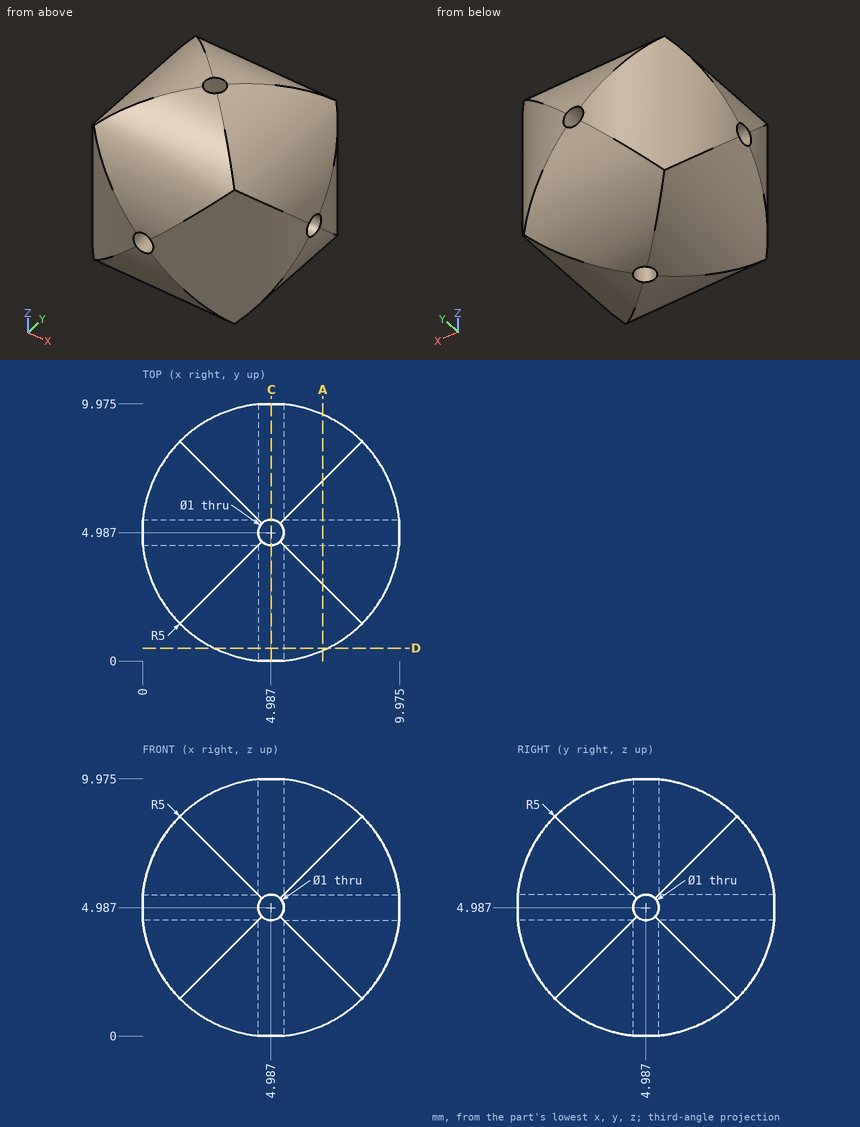
Geometry check sheet. Reference: drawing and pictorial views, mm from the part's lowest x, y, z. Coordinates: 2 decimals unless noted, no trailing zeros. Write each loop counter-clockwise with the first axis right and the second up, starting at its lowest first coordinate (ties: lowest second). Pieces come first, ordered by that corner, then holes. Notation, with made-up numbers: M -1.5,9.5 L 35.5,9.5 A18 cw 35.5,25.5 Z; hole C 16.25,50.5 d8. An arc over 180 degrees is marked long. Use one line per item in the form item = value.
Item 1: Sectioned sample at C-C, the plane x = 5. Record the cut outline in (y, z).
Answer below:
outline = M 0.01,4.49 A5 ccw 4.49,0.01 L 4.49,4.49 Z; M 0.01,5.49 L 4.49,5.49 L 4.49,9.96 A5 ccw Z; M 5.49,0.01 A5 ccw 9.96,4.49 L 5.49,4.49 Z; M 5.49,5.49 L 9.96,5.49 A5 ccw 5.49,9.96 Z
Item 2: Gauge pin test, flat ends, axial feed: pin 1 Ø1 at (x, y) = (2.5, 5) entering from -Z; pin 2 Ø3 at (x, z) = (5.5, 7.5) entering from -Y; pin 3 Ø3 at (x, y) = (5.5, 7.5) entering from +Z. Record the tip position at first contact, or that the pin passes through.
Answer below:
pin_1 = 0.4
pin_2 = 0.09
pin_3 = 9.88
Item 3: Material ranges on L1, parallel to Z at x = 5.25, y = 6 (1 decimal); L2, parallel to Z at x = 3.5, y = 3.75 (1 decimal); L3, parallel to X at y = 3.75, z = 1.5 (1 decimal), recorded low to high. Write a range as from..to.
Answer below:
L1 = 0.1..4.6, 5.4..9.9
L2 = 0.2..9.8
L3 = 1.4..8.6
Item 4: Sectioned sample at D-D, the plane y = 0.5. Record the cut outline in (x, z).
Answer below:
outline = M 2.78,2.78 L 7.19,2.78 L 7.19,7.19 L 2.78,7.19 Z; hole C 4.99,4.99 d1
Item 5: Sectioned sample at A-A, the plane x = 7. Record the cut outline in (y, z) (1 decimal).
Answer below:
outline = M 0.4,3 A5 ccw 3,0.4 L 7,0.4 A5 ccw 9.6,3 L 9.6,7 A5 ccw 7,9.6 L 3,9.6 A5 ccw 0.4,7 Z; hole C 5,5 d1
